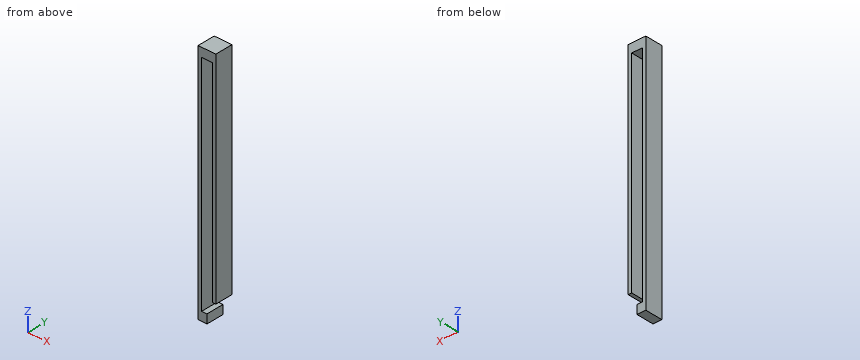
```python
from build123d import *

# Parameters (mm, degrees)
SKETCH1_W           = 10
SKETCH1_H           = 136
BOSS_EXTRUDE1_DEPTH = 10
CUT_EXTRUDE1_DEPTH  = 10
SKETCH4_W           = 2
SKETCH4_H           = 12
CUT_EXTRUDE3_DEPTH  = 10


with BuildPart() as part:
    # Sketch1 → Boss-Extrude1 (new body)
    with BuildSketch(Plane(origin=(0, 0, 0), x_dir=(1, 0, 0), z_dir=(0, 1, 0))):
        Rectangle(SKETCH1_W, SKETCH1_H)
    extrude(amount=BOSS_EXTRUDE1_DEPTH)

    # Sketch2 → Cut-Extrude1 (cut)
    with BuildSketch(Plane(origin=(0, 0, 0), x_dir=(1, 0, 0), z_dir=(0, 1, 0))):
        Polygon((0, -63), (-3, -63), (-3, 63), (0, 63), (0, 68), (3, 68), (3, 63), (3, -63), align=None)
    extrude(amount=CUT_EXTRUDE1_DEPTH, mode=Mode.SUBTRACT)

    # Sketch4 → Cut-Extrude3 (cut)
    with BuildSketch(Plane(origin=(0, 10, 0), x_dir=(1, 0, 0), z_dir=(0, 1, 0))):
        with Locations((4, 62)):
            Rectangle(SKETCH4_W, SKETCH4_H)
    extrude(amount=-CUT_EXTRUDE3_DEPTH, mode=Mode.SUBTRACT)


solid = part.part
```
Verification items for the finished model (mm, model axes). Round coordinates to 2 decimals unless told otherwise and drop trailing zeros. Loops run counter-clockwise (first coordinate to the right, second up) from the corner with the lowest first, then second, coordinate; pieces in that order, holes last. Notation, with made-up numbers: (74.25, 60) -> (88.25, 60) arc R21 cw to (88.25, 74) -> close; hole circle Ø11 at (-3, 10.5). An arc over 180 degrees is marked (long way). Answer as a JSON object with one key per item and string values.
Q1. Section check B-B (y = 7.5). Record the boundary of the cut face in (x, z).
Data:
{"outline": "(-5, -68) -> (0, -68) -> (0, -63) -> (-3, -63) -> (-3, 63) -> (3, 63) -> (3, -56) -> (5, -56) -> (5, 68) -> (-5, 68) -> close"}
Q2. Section check A-A (z = -16). Record the boundary of the cut face in (x, y), then the cut area to 3 significant figures.
Data:
{"outline": "(-5, 0) -> (-3, 0) -> (-3, 10) -> (-5, 10) -> close; (3, 0) -> (5, 0) -> (5, 10) -> (3, 10) -> close", "area": "40.0 mm2"}
Q3. Scan lines: line 1 (X direction, y = 5.25, z = 53); line 2 (Z direction, x = -1, y = 0.75); line 3 (Z direction, x = 2.5, y = 6.25). Record each from-to range of solid material in increasing order. Write a range as from..to.
Data:
{"line 1": "x = -5..-3, 3..5", "line 2": "z = -68..-63, 63..68", "line 3": "z = 63..68"}
Q4. Go/stop test with flat-tipped pins: P1, Ø1.5, axis at y = 2.5, z = -66.5, coming from the +X side; P2, Ø0.6, axis at x = 3.5, y = 4.5, coming from the -Z side. Record where each tip stops, or that it passes through.
Data:
{"P1": "stops at x = 0", "P2": "stops at z = -56"}
